```python
from build123d import *

# Parameters (mm, degrees)
SKETCH_1_W             = 5
SKETCH_1_H             = 5
EXTRUDE_1_DEPTH        = 7
SKETCH_2_R             = 2
EXTRUDE_2_DEPTH        = 1.5
SKETCH_3_R             = 1.5
EXTRUDE_3_DEPTH        = 9
HOLE_WIZARD_M3_2_D     = 2.5
HOLE_WIZARD_M3_2_DEPTH = 7.5
HOLE_WIZARD_M3_2_TIP   = 0.751075774


with BuildPart() as part:
    # 草图1 → 凸台-拉伸1 (new body)
    with BuildSketch(Plane.XY):
        with Locations((2.5, 2.5)):
            Rectangle(SKETCH_1_W, SKETCH_1_H)
    extrude(amount=EXTRUDE_1_DEPTH)

    # 草图2 → 凸台-拉伸2 (add)
    with BuildSketch(Plane.XY.offset(7)):
        with Locations((2.5, 2.5)):
            Circle(SKETCH_2_R)
    extrude(amount=EXTRUDE_2_DEPTH)

    # 草图3 → 凸台-拉伸3 (add)
    with BuildSketch(Plane.XY.offset(8.5)):
        with Locations((2.5, 2.5)):
            Circle(SKETCH_3_R)
    extrude(amount=EXTRUDE_3_DEPTH)

    # M3 螺纹孔2
    with Locations(Plane(origin=(5, 2.5, 3.5), x_dir=(0, 0, 1), z_dir=(1, 0, 0))):
        with Locations((0, 0)):
            Hole(HOLE_WIZARD_M3_2_D / 2, depth=HOLE_WIZARD_M3_2_DEPTH)
            with Locations((0, 0, -(HOLE_WIZARD_M3_2_DEPTH + HOLE_WIZARD_M3_2_TIP / 2))):  # 118° drill point
                Cone(0, HOLE_WIZARD_M3_2_D / 2, HOLE_WIZARD_M3_2_TIP, mode=Mode.SUBTRACT)


solid = part.part
```
Geometry: final body of the model. Coordinates: model frame, mm. A direction names the side the tool comes from. Round coordinates to 2 decimals unless told otherwise and drop trailing zeros. Order: outer loops, then holes, each group sorted by start corner. A loop starts at its lowest first (then second) coordinate and runs counter-clockwise, first axis right, second up. Notation, with made-up numbers: M -0.75,14 L 30.25,14 A13 ccw 30.25,24 Z; hole C -23,67 d9. An arc over 180 degrees is marked long. Use one line per item in the form item = value. Start each with the question number.
Q1. Cut plane A-A (z = 3.5). Return loops of the section in (x, y), and give its area (3 significant figures).
Q2. Pin query (flat end, axial travel): pin 1 Ø2 at (y, z) = (2.5, 3.5) entering from +X; pin 2 Ø1.5 at (x, z) = (3.5, 9.5) entering from +Y; pin 3 Ø2 at (y, z) = (3.5, 3.5) entering from -X; pin 4 Ø2 at (y, z) = (3, 14.5) entering from -X. Return the tip coordinate at first contact, or that it passes through.
Q3. Cut plane B-B (y = 2.5). Return loops of the section in (x, z).
Q4. Access query for faces 4 (the face through (2.175, 1.036, 12.937)), 5 (the face through (2, 5, 3)). Directions: +Z, -Z, +X, -X, +Y, -Y. A direction counts if a zero-diameter tool reaches every point of the face in a straight line with its end or side. Return the directions, or none.
Q5. Mould query, pull axis Z, two halves, no side actions, for faces 1 (the face through (2.066, 0.548, 7.74)), 2 (the face through (2.46, 2.12, 2.31)), 3 (the face through (0.2, 2.5, 7)). Classes: +Z half, -Z half, draft (parallel to the pull), parting line (faces both ways), or undercut.
Q6. Cut plane C-C (x = 2.5). Return loops of the section in (y, z), and give its area (3 significant figures).
Q7. Material intervals for line 1 (Y direction, x = 2.05, z = 3.5); line 2 (Z direction, x = 2.3, y = 2.6); line 3 (Z direction, x = 2.5, y = 0.6), sorted ascending. Write a range as [from, to].
Q8. Cut plane D-D (z = 8.25). Return loops of the section in (x, y), and give its area (3 significant figures).
Geometry results:
q1.outline = M 0,0 L 5,0 L 5,1.25 L 0,1.25 Z; M 0,3.75 L 5,3.75 L 5,5 L 0,5 Z
q1.area = 12.5 mm^2
q2.pin_1 = through
q2.pin_2 = 3.98
q2.pin_3 = 0
q2.pin_4 = 1
q3.outline = M 0,0 L 5,0 L 5,2.25 L 0,2.25 Z; M 0,4.75 L 5,4.75 L 5,7 L 4.5,7 L 4.5,8.5 L 4,8.5 L 4,17.5 L 1,17.5 L 1,8.5 L 0.5,8.5 L 0.5,7 L 0,7 Z
q4.face_4 = +Z
q4.face_5 = +Z, -Z, +X, -X, +Y
q5.face_1 = draft
q5.face_2 = undercut
q5.face_3 = +Z half
q6.outline = M 0,0 L 5,0 L 5,7 L 4.5,7 L 4.5,8.5 L 4,8.5 L 4,17.5 L 1,17.5 L 1,8.5 L 0.5,8.5 L 0.5,7 L 0,7 Z; hole C 2.5,3.5 d2.5
q6.area = 63.1 mm^2
q7.line_1 = [0, 1.25], [3.75, 5]
q7.line_2 = [0, 2.25], [4.75, 17.5]
q7.line_3 = [0, 8.5]
q8.outline = C 2.5,2.5 d4
q8.area = 12.6 mm^2
